Input: part model. Units: mm. Frame: model coordinates. Give positions to 0.01 mm unless a question says otherwise; leave off trailing zeros. Loops run counter-clockwise (first coordinate to the right, second up) from the corner with the lowest first, then second, coordinate; pieces in that order, holes last. Notation, with made-up numbers: (53.5, 64) -> (98.5, 64) arc R22 cw to (98.5, 87) -> close; hole circle Ø7 at (45.25, 62.25). An arc over 180 degrees is marked (long way). Answer as a JSON object with one key per item and string values. Group by question number.
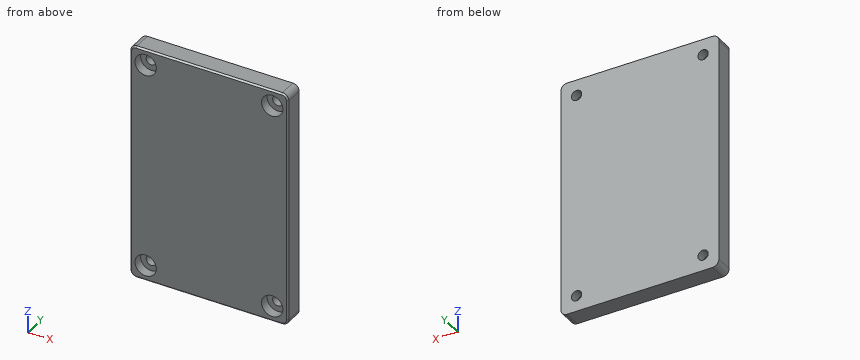
Autodesk Inventor part; units mm, degrees
ref_plane "YZ Plane" through (0, 0, 0) normal (1, 0, 0) x (0, 1, 0)
ref_plane "XZ Plane" through (0, 0, 0) normal (0, 1, 0) x (-1, 0, 0)
ref_plane "XY Plane" through (0, 0, 0) normal (0, 0, 1) x (1, 0, 0)
sketch "Sketch1" plane through (0, 0, 0) normal (0, 1, 0) x (-1, 0, 0)
  line L0 (-50, 75) -> (50, 75)
  line L1 (50, 75) -> (50, -75)
  line L2 (50, -75) -> (-50, -75)
  line L3 (-50, -75) -> (-50, 75)
  line L4 (-50, 75) -> (50, -75) construction
  line L5 (50, 75) -> (-50, -75) construction
  point P0 (0, 0)
  dimension "d0" = 150
  dimension "d1" = 100
extrude "Extrusion1" add sketch "Sketch1" along normal blind 12
sketch "Sketch3" plane through (0, 0, 0) normal (0, -1, 0) x (1, 0, 0)
  circle A0 centre (40, 65) radius 7
  circle A1 centre (40, 65) radius 3.25
  line L0 (50, 75) -> (50, -75)
  line L1 (-50, 75) -> (50, 75)
  circle A2 centre (40, -65) radius 3.25
  circle A3 centre (40, -65) radius 7
  circle A4 centre (-40, 65) radius 3.25
  circle A5 centre (-40, 65) radius 7
  circle A6 centre (-40, -65) radius 3.25
  circle A7 centre (-40, -65) radius 7
  point P0 (0, 0)
  dimension "d4" = 14
  dimension "d5" = 6.5
  dimension "d6" = 10
  dimension "d7" = 10
  dimension "d10" = 130
  dimension "d13" = 80
hole "Hole1" at (40, 0, 65) at (40, 0, -65) at (-40, 0, 65) at (-40, 0, -65) direction (0, 1, 0) diameter 6.5 end through all counterbore diameter 13.5 counterbore depth 6
fillet "Fillet1" radius 4 4 edges at (50, 6, 75) (50, 6, -75) (-50, 6, -75) (-50, 6, 75)
chamfer "Chamfer3" distance 1 angle 45 8 edges at (0, 0, 75) (48.8284, 0, 73.8284) (50, 0, 0) (48.8284, 0, -73.8284) (0, 0, -75) (-48.8284, 0, -73.8284) (-50, 0, 0) (-48.8284, 0, 73.8284)
properties part number "PCB_Cover"
Q1. Section A-A on x = 40. Return the cut outline in (y, z).
Q2. Section C-C on z = -65. Return the cut outline in (x, y).
Q3. Ray query, probe 1 along Z at (x, y) = (-40, 1.3); probe 2 along Z at (x, y) = (-40, 7.3); probe 3 along X at (y, z) = (2.15, -65). Return the intervals inside material, ascending.
Q4. Pin query (flat end, axial travel): pin 1 Ø7 at (x, z) = (37, -65.5) entering from -Y. Return the tip coordinate at first contact, or that it passes through.
Q5. Section B-B on y = 4. Return the cut outline in (x, z), then the cut area to 3 significant figures.
Numbers:
{
 "1": {"outline": "(0, -74) -> (1, -75) -> (12, -75) -> (12, -68.25) -> (6, -68.25) -> (6, -71.75) -> (0, -71.75) -> close; (0, -58.25) -> (6, -58.25) -> (6, -61.75) -> (12, -61.75) -> (12, 61.75) -> (6, 61.75) -> (6, 58.25) -> (0, 58.25) -> close; (0, 71.75) -> (6, 71.75) -> (6, 68.25) -> (12, 68.25) -> (12, 75) -> (1, 75) -> (0, 74) -> close"},
 "2": {"outline": "(-50, 1) -> (-49, 0) -> (-46.75, 0) -> (-46.75, 6) -> (-43.25, 6) -> (-43.25, 12) -> (-50, 12) -> close; (-36.75, 6) -> (-33.25, 6) -> (-33.25, 0) -> (33.25, 0) -> (33.25, 6) -> (36.75, 6) -> (36.75, 12) -> (-36.75, 12) -> close; (43.25, 6) -> (46.75, 6) -> (46.75, 0) -> (49, 0) -> (50, 1) -> (50, 12) -> (43.25, 12) -> close"},
 "3": {"probe 1": "z = -75 to -71.75, -58.25 to 58.25, 71.75 to 75", "probe 2": "z = -75 to -68.25, -61.75 to 61.75, 68.25 to 75", "probe 3": "x = -50 to -46.75, -33.25 to 33.25, 46.75 to 50"},
 "4": {"pin 1": "stops at y = 6"},
 "5": {"outline": "(-50, -71) arc R4 ccw to (-46, -75) -> (46, -75) arc R4 ccw to (50, -71) -> (50, 71) arc R4 ccw to (46, 75) -> (-46, 75) arc R4 ccw to (-50, 71) -> close; hole circle Ø13.5 at (-40, -65); hole circle Ø13.5 at (-40, 65); hole circle Ø13.5 at (40, -65); hole circle Ø13.5 at (40, 65)", "area": "14,400 mm²"}
}
